Geometry: final body of the model. Coordinates: model frame, mm. A direction names the side the tool comes from. Give positions to 0.01 mm unless a question says otherwise; leave off trailing zeros. Write each loop counter-clockwise with the first axis right and the second up, starting at its lowest first coordinate (ties: lowest second). Pieces come first, ordered by that corner, then holes.
from build123d import *

# Parameters (mm, degrees)
CROQUIS1_R              = 6.5
SALIENTE_EXTRUIR1_DEPTH = 1.2
CROQUIS2_R              = 5
SALIENTE_EXTRUIR2_DEPTH = 3
CROQUIS3_R              = 1.8
CORTAR_EXTRUIR1_DEPTH   = 3
CORTAR_EXTRUIR2_REACH   = 6.2
CROQUIS4_R              = 1.9
CROQUIS5_R              = 6.5
SALIENTE_EXTRUIR3_DEPTH = 2.5
CORTAR_EXTRUIR3_DEPTH   = 2.5


with BuildPart() as part:
    # Croquis1 → Saliente-Extruir1 (new body)
    with BuildSketch(Plane(origin=(0, 0, 0), x_dir=(1, 0, 0), z_dir=(0, 1, 0))):
        Circle(CROQUIS1_R)
    extrude(amount=SALIENTE_EXTRUIR1_DEPTH)

    # Croquis2 → Saliente-Extruir2 (add)
    with BuildSketch(Plane(origin=(0, 1.2, 0), x_dir=(1, 0, 0), z_dir=(0, 1, 0))):
        Circle(CROQUIS2_R)
    extrude(amount=SALIENTE_EXTRUIR2_DEPTH)

    # Croquis3 → Cortar-Extruir1 (cut)
    with BuildSketch(Plane(origin=(0, 4.2, 0), x_dir=(1, 0, 0), z_dir=(0, 1, 0))):
        Circle(CROQUIS3_R)
    extrude(amount=-CORTAR_EXTRUIR1_DEPTH, mode=Mode.SUBTRACT)

    # Croquis4 → Cortar-Extruir2 (cut, up to next)
    with BuildSketch(Plane.XZ, mode=Mode.PRIVATE) as cortar_extruir2_sk1:
        Circle(CROQUIS4_R)
    cortar_extruir2_tool1 = extrude(cortar_extruir2_sk1.sketch, amount=-CORTAR_EXTRUIR2_REACH, mode=Mode.PRIVATE) & part.part
    add(cortar_extruir2_tool1.solids().sort_by_distance((0, 0, 0))[0], mode=Mode.SUBTRACT)

    # Croquis5 → Saliente-Extruir3 (add)
    with BuildSketch(Plane.XZ):
        Circle(CROQUIS5_R)
    extrude(amount=SALIENTE_EXTRUIR3_DEPTH)

    # Croquis6 → Cortar-Extruir3 (cut)
    with BuildSketch(Plane.XZ.offset(2.5)):
        Polygon((-3.300733133, 1.228207686), (-2.714025623, -2.244414901), (0.586707509, -3.472622587), (3.300733133, -1.228207686), (2.714025623, 2.244414901), (-0.586707509, 3.472622587), align=None)
    extrude(amount=-CORTAR_EXTRUIR3_DEPTH, mode=Mode.SUBTRACT)


solid = part.part
Q1. Pin query (flat end, axial travel): P1, Ø4, axis at y = -1.5, z = 5, coming from the +X side; P2, Ø1, axis at x = 0.5, y = 1.5, coming from the -Z side; P3, Ø1, axis at x = 4.5, y = 1.5, coming from the -Z side; P4, Ø4, axis at y = -0.5, z = 3, coming from the -X side. Return the tip coordinate at first contact, or that it passes through.
Filled sheet:
P1: stops at x = 5.77
P2: stops at z = -6.5
P3: stops at z = -5.04
P4: stops at x = -6.42
Q2. Pull-direction query (Z, two-part tool) for faces 1 (the flat face through (2, 1.2, 5)), 2 (the flat face through (1.4, 0, -1.5)), 3 (the flat face through (-3.011, -1.268, -0.484)), 4 (the cylindrical face through (-5.158, -0.624, -3.955)); classes: released by +Z, released by -Z, zero draft, split by the parting line, or undercut.
Filled sheet:
face 1: zero draft
face 2: undercut
face 3: undercut
face 4: split by the parting line
Q3. Access query for faces 5 (the flat face through (-1.92, -1.27, 2.37)), 6 (the cylindrical face through (-1.08, 2.68, 4.88)), 7 (the flat face through (-0.1, 4.2, 2.2)). Directions: +Z, -Z, +X, -X, +Y, -Y. A direction counts if a zero-diameter tool reaches every point of the face in a straight line with its end or side. Return the directions, or none.
Filled sheet:
face 5: -Y
face 6: +Y
face 7: +Z, -Z, +X, -X, +Y
Q4. Ray query, line 1 along Z through (x, y) = (0, 3.1); line 2 along Z through (x, y) = (-2.5, -0.5); line 3 along X through (y, z) = (2.25, 1.5). Return the intervals inside material, ascending.
Filled sheet:
line 1: z = -5 to -1.9, 1.9 to 5
line 2: z = -6 to -2.32, 1.89 to 6
line 3: x = -4.77 to -1.17, 1.17 to 4.77
Q5. Section D-D on z = 3. Output: boundary loops of the cut face in (x, y).
Filled sheet:
outline: (-5.77, -2.5) - (-1.16, -2.5) - (-1.16, 0) - (0.68, 0) - (0.68, -2.5) - (5.77, -2.5) - (5.77, 1.2) - (4, 1.2) - (4, 4.2) - (-4, 4.2) - (-4, 1.2) - (-5.77, 1.2) - close
Q6. Section A-A on y = -0.25. Output: boundary loops of the cut face in (x, z).
Filled sheet:
outline: circle Ø13 at (0, 0); hole (-3.3, 1.23) - (-2.71, -2.24) - (0.59, -3.47) - (3.3, -1.23) - (2.71, 2.24) - (-0.59, 3.47) - close
Q7. Section C-C on x = 0. Output: boundary loops of the cut face in (y, z), plus the area to 3 significant figures.
Filled sheet:
outline: (-2.5, -6.5) - (1.2, -6.5) - (1.2, -5) - (4.2, -5) - (4.2, -1.9) - (0, -1.9) - (0, -3.25) - (-2.5, -3.25) - close; (-2.5, 3.25) - (0, 3.25) - (0, 1.9) - (4.2, 1.9) - (4.2, 5) - (1.2, 5) - (1.2, 6.5) - (-2.5, 6.5) - close
area: 45.9 mm2
Q8. Section B-B on z = 0. Output: boundary loops of the cut face in (x, y).
Filled sheet:
outline: (-6.5, -2.5) - (-3.09, -2.5) - (-3.09, 0) - (-1.9, 0) - (-1.9, 4.2) - (-5, 4.2) - (-5, 1.2) - (-6.5, 1.2) - close; (1.9, 0) - (3.09, 0) - (3.09, -2.5) - (6.5, -2.5) - (6.5, 1.2) - (5, 1.2) - (5, 4.2) - (1.9, 4.2) - close
